Geometry: final body of the model. Coordinates: model frame, mm. A direction names the side the tool comes from. Give positions to 0.01 mm unless a question says otherwise; leave off trailing zeros. Write each loop counter-clockwise with the first axis right and the second up, starting at its lowest first coordinate (ties: lowest second). Pieces come first, ordered by that corner, then holes.
from build123d import *

# Parameters (mm, degrees)
SKETCH4_W           = 62
SKETCH4_H           = 62
SKETCH4_R           = 3
SKETCH4_R_2         = 2.5
SKETCH4_R_3         = 2.625
BOSS_EXTRUDE2_DEPTH = 5
SKETCH5_W           = 10.4
SKETCH5_H           = 1.2
SKETCH5_W_2         = 1.2
SKETCH5_H_2         = 10.4
CUT_EXTRUDE1_DEPTH  = 2
FILLET1_R           = 10
SKETCH6_W           = 10
SKETCH6_H           = 11
BOSS_EXTRUDE3_DEPTH = 4
SKETCH7_R           = 2.6
CUT_EXTRUDE2_DEPTH  = 9
CHAMFER1_SIZE       = 1
FILLET2_R           = 2


with BuildPart() as part:
    # Sketch3 → Revolve1 (revolve)
    with BuildSketch(Plane.XY, mode=Mode.PRIVATE) as revolve1_sk:
        with BuildLine():
            Line((0, 0), (2.7, 0))
            Line((2.7, 0), (2.233206222, 1.282505364))
            ThreePointArc((2.233206222, 1.282505364), (1.26348021, 0.413869711), (0, 0.1))
            Line((0, 0.1), (0, 0))
        make_face()
    revolve(revolve1_sk.sketch.rotate(Axis((0, 0.1, 0), (0, -1, 0)), 90), axis=Axis((0, 0.1, 0), (0, -1, 0)))

    # Sketch4 → Boss-Extrude2 (add)
    with BuildSketch(Plane.XZ):
        Rectangle(SKETCH4_W, SKETCH4_H)
        with Locations(Location((17.5, 0, 0), (0, 0, 270))):
            Circle(SKETCH4_R, mode=Mode.SUBTRACT)
        with Locations(Location((0, 17.5, 0), (0, 0, 270))):
            Circle(SKETCH4_R, mode=Mode.SUBTRACT)
        with Locations(Location((-15, -15, 0), (0, 0, 270))):
            Circle(SKETCH4_R_2, mode=Mode.SUBTRACT)
        with Locations(Location((0, 25.5, 0), (0, 0, 270))):
            Circle(SKETCH4_R_3, mode=Mode.SUBTRACT)
        with Locations(Location((25.5, 0, 0), (0, 0, 270))):
            Circle(SKETCH4_R_3, mode=Mode.SUBTRACT)
    extrude(amount=BOSS_EXTRUDE2_DEPTH)

    # Sketch5 → Cut-Extrude1 (cut)
    with BuildSketch(Plane.XZ.offset(5)):
        with Locations((0, 17.5)):
            Rectangle(SKETCH5_W, SKETCH5_H)
        with Locations((17.5, 0)):
            Rectangle(SKETCH5_W_2, SKETCH5_H_2)
        Polygon((-18.252691193, -10.898780669), (-10.898780669, -18.252691193), (-11.747308807, -19.101219331), (-19.101219331, -11.747308807), align=None)
    extrude(amount=-CUT_EXTRUDE1_DEPTH, mode=Mode.SUBTRACT)

    # Fillet1
    fillet1_edges = [part.edges().sort_by_distance(p)[0] for p in [
        (31, -2.5, -31),
        (31, -2.5, 31),
        (-31, -2.5, 31),
        (-31, -2.5, -31),
    ]]
    fillet(fillet1_edges, radius=FILLET1_R)

    # Sketch6 → Boss-Extrude3 (add)
    with BuildSketch(Plane(origin=(0, 0, 0), x_dir=(1, 0, 0), z_dir=(0, 1, 0))):
        with Locations((-26, 0)):
            Rectangle(SKETCH6_W, SKETCH6_H)
    extrude(amount=BOSS_EXTRUDE3_DEPTH)

    # Sketch7 → Cut-Extrude2 (cut)
    with BuildSketch(Plane.ZY.offset(31)):
        with Locations((0, -0.5)):
            Circle(SKETCH7_R)
    extrude(amount=-CUT_EXTRUDE2_DEPTH, mode=Mode.SUBTRACT)

    # Chamfer1
    chamfer1_edges = [part.edges().sort_by_distance(p)[0] for p in [
        (-31, -0.5, -2.6),
    ]]
    chamfer(chamfer1_edges, length=CHAMFER1_SIZE)

    # Fillet2
    fillet2_edges = [part.edges().sort_by_distance(p)[0] for p in [
        (-26, 0, 5.5),
        (-21, 0, 0),
        (-21, 2, 5.5),
        (-26, 0, -5.5),
        (-21, 2, -5.5),
        (-26, 4, 5.5),
        (-21, 4, 0),
        (-26, 4, -5.5),
    ]]
    fillet(fillet2_edges, radius=FILLET2_R - 0.0001)  # a hair under: the kernel refuses the full size


solid = part.part
Q1. Pull-direction query (X, two-part tool) for faces 4 (the cylindrical face through (27.99, -2.54, -28.15)), 5 (the cylindrical face through (-26.056, 2.078, -0.338)), 6 (the flat face through (16.9, -4, -4)), 7 (the cylindrical face through (-28.15, -2.54, -27.99)); classes: released by +X, released by -X, zero draft, split by the parting line, or undercut.
Filled sheet:
face 4: released by +X
face 5: zero draft
face 6: undercut
face 7: released by -X
Q2. Pin query (flat end, axial travel): P1, Ø5, axis at x = -5, z = 15, coming from the +Y side; P2, Ø0.6, axis at x = 17.5, z = 4.5, coming from the -Y side. Return the tip coordinate at first contact, or that it passes through.
Filled sheet:
P1: stops at y = 0
P2: stops at y = -3
Q3. Section B-B on x = -15. Output: boundary loops of the cut face in (y, z), plus the area to 3 significant figures.
Filled sheet:
outline: (-5, -31) - (0, -31) - (0, -17.5) - (-5, -17.5) - close; (-5, -12.5) - (0, -12.5) - (0, 31) - (-5, 31) - close
area: 285 mm2
Q4. Access query for faces 1 (the flat face through (-11.89, -4.01, -17.26)), 2 (the flat face through (-22, 0, 0)), 3 (the cylindrical face through (0.115, -2.465, 28.122)). Directions: +Z, -Z, +X, -X, +Y, -Y. A direction counts if a zero-diameter tool reaches every point of the face in a straight line with its end or side. Return the directions, or none.
Filled sheet:
face 1: -Y
face 2: -X
face 3: +Y, -Y
Q5. Ray query, line 1 along Z through (x, y) = (-15, -1.35); line 2 along X through (y, z) = (-2.05, 0) (3 decimals); line 3 along X through (y, z) = (-2.1, 17.5). Return the intervals inside material, ascending.
Filled sheet:
line 1: z = -31 to -17.5, -12.5 to 31
line 2: x = -22 to 14.5, 20.5 to 22.875, 28.125 to 31
line 3: x = -31 to -3, 3 to 31
Q6. Section D-D on z = -1.5. Count the separate pieces of the cut face and the enclosed holes in it, plus the area to 3 significant figures.
Filled sheet:
separate pieces: 3
enclosed holes: 0
area: 266 mm2
Q7. Section C-C on x = 0. Output: boundary loops of the cut face in (y, z) (1 decimal), plus the area to 3 significant figures.
Filled sheet:
outline: (-5, -31) - (0, -31) - (0, -2.7) - (1.3, -2.2) arc R2.7 cw to (1.3, 2.2) - (0, 2.7) - (0, 14.5) - (-5, 14.5) - close; (-5, 20.5) - (0, 20.5) - (0, 22.9) - (-5, 22.9) - close; (-5, 28.1) - (0, 28.1) - (0, 31) - (-5, 31) - close
area: 256 mm2
Q8. Section A-A on z = -15. Output: boundary loops of the cut face in (x, y), plus the area to 3 significant figures.
Filled sheet:
outline: (-31, -5) - (-17.5, -5) - (-17.5, 0) - (-31, 0) - close; (-12.5, -5) - (31, -5) - (31, 0) - (-12.5, 0) - close
area: 285 mm2
